```python
from build123d import *

# Parameters (mm, degrees)
BOSS_EXTRUDE1_DEPTH = 7.5
SKETCH2_R           = 3.5
CUT_EXTRUDE1_DEPTH  = 4.4
FILLET1_START       = -4.4
FILLET1_DEPTH       = 5.4
SKETCH3_R           = 1.9
BOSS_EXTRUDE2_DEPTH = 7.5
CUT_EXTRUDE2_REACH  = 21.056
SKETCH7_R           = 1
CUT_EXTRUDE3_DEPTH  = 7.5
CUT_EXTRUDE4_DEPTH  = 6


with BuildPart() as part:
    # Sketch1 → Boss-Extrude1 (new body)
    with BuildSketch(Plane(origin=(0, 0, 0), x_dir=(0, 0, -1), z_dir=(1, 0, 0))):
        with BuildLine():
            Line((12.5, -3.5), (7.528802268, -3.5))
            Line((7.528802268, -3.5), (-12.5, -2.5))
            Line((-12.5, -2.5), (-15.372715308, -1.549625261))
            ThreePointArc((-15.372715308, -1.549625261), (-15.869210997, -1.185856004), (-16.058629018, -0.600230821))
            Line((-16.058629018, -0.600230821), (-16.058629018, 0.344074306))
            ThreePointArc((-16.058629018, 0.344074306), (-15.891200042, 0.897992613), (-15.444978036, 1.26642697))
            Line((-15.444978036, 1.26642697), (-12.5, 2.5))
            Line((-12.5, 2.5), (3.930719529, 3.5))
            Line((3.930719529, 3.5), (12.5, 3.5))
            ThreePointArc((12.5, 3.5), (16, 0), (12.5, -3.5))
        make_face()
    extrude(amount=-BOSS_EXTRUDE1_DEPTH)

    # Sketch2 → Cut-Extrude1 (cut)
    with BuildSketch(Plane(origin=(0, 0, 0), x_dir=(0, 0, -1), z_dir=(1, 0, 0))):
        with Locations((12.5, 0)):
            Circle(SKETCH2_R)
    extrude(amount=-CUT_EXTRUDE1_DEPTH, mode=Mode.SUBTRACT)

    # Fillet1: read off the stored shape, not the designer's step
    # Fillet1 outline → Fillet1 (cut)
    with BuildSketch(Plane.YZ.offset(FILLET1_START)):
        with BuildLine():
            ThreePointArc((3.5, -9.854248689), (3.176776695, -10.321955862), (2.625, -10.184967603))
            ThreePointArc((2.625, -10.184967603), (3.273950213, -11.262563133), (3.5, -12.5))
            Line((3.5, -12.5), (3.5, -9.854248689))
        make_face()
        with BuildLine():
            ThreePointArc((-2.625, -10.184967603), (-3.176776695, -10.321955862), (-3.5, -9.854248689))
            Line((-3.5, -9.854248689), (-3.5, -12.5))
            ThreePointArc((-3.5, -12.5), (-3.273950213, -11.262563133), (-2.625, -10.184967603))
        make_face()
    extrude(amount=FILLET1_DEPTH, mode=Mode.SUBTRACT)

    # Sketch3 → Boss-Extrude2 (add)
    with BuildSketch(Plane.ZY.offset(7.5)):
        with Locations(Location((-12.5, 0, 0), (0, 0, 180))):
            Circle(SKETCH3_R)
    extrude(amount=-BOSS_EXTRUDE2_DEPTH)

    # Cut-Extrude2: up to this plane
    cut_extrude2_end = Plane(origin=(-7.5, -3.116332783, 0.155592568), z_dir=(0, 0.9987559179882337, -0.04986598322986022))
    # Sketch4 → Cut-Extrude2 (cut, up to the surface)
    with BuildSketch(Plane(origin=(0, 3.5, 0), x_dir=(1, 0, 0), z_dir=(0, 1, 0)), mode=Mode.PRIVATE) as cut_extrude2_sk1:
        Polygon((-7.5, -16.058629018), (-7.5, 3.930719529), (-6, -16.058629018), align=None)
    cut_extrude2_tool1 = split(extrude(cut_extrude2_sk1.sketch, amount=-CUT_EXTRUDE2_REACH, mode=Mode.PRIVATE), bisect_by=cut_extrude2_end, keep=Keep.BOTH, mode=Mode.PRIVATE)
    add(cut_extrude2_tool1.solids().sort_by_distance((-7, 3.5, 9.395513))[0], mode=Mode.SUBTRACT)

    # Sketch7 → Cut-Extrude3 (cut)
    with BuildSketch(Plane.ZY.offset(7.5)):
        with Locations((-12.5, 0)):
            Circle(SKETCH7_R)
        with Locations(Location((12.5, 0, 0), (0, 0, 180))):
            Circle(SKETCH7_R)
    extrude(amount=-CUT_EXTRUDE3_DEPTH, mode=Mode.SUBTRACT)

    # Sketch8 → Cut-Extrude4 (cut)
    with BuildSketch(Plane.ZY.offset(7.5)):
        Polygon((-11, 0), (-11.75, 1.299038106), (-13.25, 1.299038106), (-14, 0), (-13.25, -1.299038106), (-11.75, -1.299038106), align=None)
        Polygon((14, 0), (13.25, 1.299038106), (11.75, 1.299038106), (11, 0), (11.75, -1.299038106), (13.25, -1.299038106), align=None)
    extrude(amount=-CUT_EXTRUDE4_DEPTH, mode=Mode.SUBTRACT)


solid = part.part
```
Build history of the part. All positions in model axes, mm. A direction names the side the tool comes from. Round coordinates to 2 decimals unless told otherwise and drop trailing zeros. Write each loop counter-clockwise with the first axis right and the second up, starting at its lowest first coordinate (ties: lowest second). Pieces come first, ordered by that corner, then holes. Notation, with made-up numbers: (42.25, 6) -> (99.25, 6) arc R13 ccw to (99.25, 11) -> close; hole circle Ø9 at (84, 34.25). An arc over 180 degrees is marked (long way). Put each result on its own line as item: value.
Item 1: Slice it at B-B, the plane z = 1. Give the cut face in (x, y), plus the area to 3 significant figures.
Here are the results:
outline: (-7.13, -3.07) -> (0, -3.07) -> (0, 3.2) -> (-7.13, 3.2) -> close
area: 44.7 mm^2
Item 2: Tool access for faces 1 (the face through (-6.927, 0.138, 3.703)), 2 (the face through (-0.8, 0, 13.5)), 3 (the face through (-4, -1.299, 12)), 4 (the face through (-2.231, -1.602, -13.521)), 5 (the face through (-2.23, 3.18, -10.32)): list every direction of +Z, -Z, +X, -X, +Y, -Y with a clear straight run to the whole face (end or side of a thin tool).
Here are the results:
face 1: +Z, -X, +Y, -Y
face 2: +X, -X
face 3: -X
face 4: +X
face 5: -Z, +X
Item 3: Slice it at A-A, the plane x = -2.5. Give the cut face in (y, z) (3 decimals), plus the area to 3 significant figures.
Here are the results:
outline: (-3.5, -9.854) arc R0.5 ccw to (-2.625, -10.185) arc R3.5 cw to (2.625, -10.185) arc R0.5 ccw to (3.5, -9.854) -> (3.5, -3.931) -> (2.5, 12.5) -> (1.266, 15.445) arc R1 ccw to (0.344, 16.059) -> (-0.6, 16.059) arc R1 ccw to (-1.55, 15.373) -> (-2.5, 12.5) -> (-3.5, -7.529) -> close; circle Ø3.8 at (0, -12.5); hole (-1.299, -13.25) -> (0, -14) -> (1.299, -13.25) -> (1.299, -11.75) -> (0, -11) -> (-1.299, -11.75) -> close; hole (-1.299, 11.75) -> (0, 11) -> (1.299, 11.75) -> (1.299, 13.25) -> (0, 14) -> (-1.299, 13.25) -> close
area: 149 mm^2
Item 4: Flat gauge pins, fed straight in: P1, Ø1.2, axis at x = -3, z = -12, coming from the -Y side; P2, Ø2.5, axis at y = 0, z = -12.5, coming from the -X side; P3, Ø1.2, axis at x = -4.5, z = 12.5, coming from the +Y side. Where does each tip first touch, or does it go through?
Here are the results:
P1: stops at y = -1.9
P2: stops at x = -1.5
P3: stops at y = 2.54
Item 5: Wall check: probe 1 along Z at (x, y) = (-2.25, 0.75); probe 2 along Z at (x, y) = (-0.25, -0.25); probe 3 along Y at (x, z) = (-0.8, -12.5). Give the ranges that are in metal, low to high. Write a range as from..to.
Here are the results:
probe 1: z = -14.25..-13.57, -11.43..-10.75, -9.08..11.43, 13.57..15.97
probe 2: z = -14.38..-13.47, -11.53..-10.62, -9.01..11.53, 13.47..16.06
probe 3: y = -1.9..-1, 1..1.9
Item 6: Two-plate mould, pull along Y, no slides. Class faces 6 (the face through (-2.983, -1.193, 15.864)), 7 (the face through (-3.89, 0.64, 13.63)), 8 (the face through (-3, 0, 16.059)), 9 (the face through (-5, -1.299, -13)): pulls with the +Y half, pulls with the -Y half, needs draft (parallel to the pull), parting line crosses it, or undercut.
Here are the results:
face 6: pulls with the -Y half
face 7: undercut
face 8: needs draft
face 9: undercut
